from build123d import *

# Parameters (mm, degrees)
SWEEP_THIN1_PROFILE_R   = 22.5
SWEEP_THIN1_PROFILE_R_2 = 15
SKETCH30_R              = 21
CUT_EXTRUDE1_DEPTH      = 10
SKETCH41_R              = 6
CUT_EXTRUDE3_DEPTH      = 90


with BuildPart() as part:
    # Sweep-Thin1: sweep along a path in Sketch1
    with BuildLine(Plane.XY) as sweep_thin1_path:
        Line((0, 0), (-220, 0))
        ThreePointArc((-220, 0), (-255.355339059, -14.644660941), (-270, -50))
        Line((-270, -50), (-270, -220))
        ThreePointArc((-270, -220), (-255.355339059, -255.355339059), (-220, -270))
        Line((-220, -270), (-200, -270))
    # Sweep-Thin1 profile (on start of the path) → Sweep-Thin1 (sweep)
    with BuildSketch(Plane(origin=(0, 0, 0), x_dir=(0, -1, 0), z_dir=(-1, 0, 0))):
        Circle(SWEEP_THIN1_PROFILE_R)
        Circle(SWEEP_THIN1_PROFILE_R_2, mode=Mode.SUBTRACT)
    sweep(path=sweep_thin1_path.line)

    # Sketch30 → Cut-Extrude1 (cut)
    with BuildSketch(Plane(origin=(-200, 0, 0), x_dir=(0, 0, -1), z_dir=(1, 0, 0))):
        with Locations((0, -270)):
            Circle(SKETCH30_R)
    extrude(amount=-CUT_EXTRUDE1_DEPTH, mode=Mode.SUBTRACT)

    # Sketch41 → Cut-Extrude3 (cut)
    with BuildSketch(Plane(origin=(0, 22.5, 0), x_dir=(1, 0, 0), z_dir=(0, 1, 0))):
        with Locations(Location((-195, 0, 0), (0, 0, 180))):
            Circle(SKETCH41_R)
    extrude(amount=-CUT_EXTRUDE3_DEPTH, mode=Mode.SUBTRACT)


solid = part.part
Can you work these out from the model? Positions are in its coordinate system, mm. A direction names the side the tool comes from. Coordinates: 2 decimals unless noted, no trailing zeros. Order: outer loops, then holes, each group sorted by start corner. A loop starts at its lowest first (then second) coordinate and runs counter-clockwise, first axis right, second up. Notation, with made-up numbers: (4.25, 55.5) - (13.25, 55.5) arc R37 cw to (13.25, 93.5) - close; hole circle Ø2 at (20, 54). An arc over 180 degrees is marked (long way). Answer as a JSON object with one key per item and string values. Group by question number.
Q1. We'd pull the mould along Z, two halves only. Please class faces 1 (the face through (-210, -284, -9)), 2 (the face through (-204.93, -290.5, 4.55)), 3 (the face through (0, 5, -15)), 4 (the face through (-248.54, -136.19, 6.76)): +Z half, -Z half, draft (parallel to the pull), parting line (faces both ways), or undercut.
Q2. Will these pins go through, and if not, where does the flat tip stop? P1, Ø2, axis at y = -160.5, z = 14, coming from the +X side; P2, Ø3, axis at y = -229.5, z = -10.5, coming from the -X side; P3, Ø21, axis at y = -265, z = -2, coming from the +X side.
Q3. On a 3-axis mill with a long thin cutter (end or side, diameter ignored), from which of +Z, -Z, +X, -X, +Y, -Y can I reach the whole of each face in a straight line? I mean faces 5 (the face through (-200, -250, -7)), 6 (the face through (-255.693, -136.19, 4.506)), 7 (the face through (-189, -18, 0)), 8 (the face through (-111.54, 14.985, 0.66)). Say none if no direction works.
Q4. Imagine slicing it at C-C (y = -202.5). Please give me the cut outline in (x, z), and give its area (3 significant figures).
Q5. Imagine slicing it at D-D (x = -227.5). Give the number of separate pieces and of enclosed holes in the cut face, and give its area (3 significant figures).
Q6. Imagine slicing it at B-B (z = 10.5). Please give me the cut outline in (x, y), and give its area (3 significant figures).
Q7. I need wall thicknesses on line 1 (X direction, y = -61.5, z = 1); line 2 (X direction, y = -69, z = 7); line 3 (Y direction, x = -33.5, z = 7.5). Which ranges of each line are inside material? Lowest first, please. Write a range as from..to.
Q8. Imagine slicing it at A-A (x = -195). Please give me the cut outline in (y, z), and give its area (3 significant figures).
Determined:
{
 "1": {"face 1": "undercut", "face 2": "undercut", "face 3": "draft", "face 4": "parting line"},
 "2": {"P1": "stops at x = -251.64", "P2": "stops at x = -290.01", "P3": "stops at x = -210"},
 "3": {"face 5": "+Z, -Z, +X, -Y", "face 6": "none", "face 7": "+Y", "face 8": "+X"},
 "4": {"outline": "circle Ø45 at (-270, 0); hole circle Ø30 at (-270, 0)", "area": "884 mm2"},
 "5": {"separate pieces": "2", "enclosed holes": "2", "area": "1,790 mm2"},
 "6": {"outline": "(-289.9, -220) arc R69.9 ccw to (-220, -289.9) - (-200, -289.9) - (-200, -288.19) - (-210, -288.19) - (-210, -280.71) - (-220, -280.71) arc R60.71 cw to (-280.71, -220) - (-280.71, -50) arc R60.71 cw to (-220, 10.71) - (0, 10.71) - (0, 19.9) - (-220, 19.9) arc R69.9 ccw to (-289.9, -50) - close; (-259.29, -220) arc R39.29 ccw to (-220, -259.29) - (-210, -259.29) - (-210, -251.81) - (-200, -251.81) - (-200, -250.1) - (-220, -250.1) arc R30.1 cw to (-250.1, -220) - (-250.1, -50) arc R30.1 cw to (-220, -19.9) - (0, -19.9) - (0, -10.71) - (-220, -10.71) arc R39.29 ccw to (-259.29, -50) - close", "area": "10,300 mm2"},
 "7": {"line 1": "x = -292.48..-284.97, -255.03..-247.52", "line 2": "x = -291.38..-283.27, -256.73..-248.62", "line 3": "y = -21.21..-12.99, 12.99..21.21"},
 "8": {"outline": "(-21.69, -6) arc R22.5 ccw to (21.69, -6) - (13.75, -6) arc R15 cw to (-13.75, -6) - close; (-21.69, 6) - (-13.75, 6) arc R15 cw to (13.75, 6) - (21.69, 6) arc R22.5 ccw to start", "area": "700 mm2"}
}
